Source: CAD feature listing. Evaluate the final solid. Frame: model axes, mm. Face numbers are marked on the shaded views. A direction names the side the tool comes from. Round coordinates to 2 decimals unless told otherwise and drop trailing zeros. Loops run counter-clockwise (first coordinate to the right, second up) from the corner with the lowest first, then second, coordinate; pieces in that order, holes last.
(1) Mould query, pull axis Y, two halves, no side actions, for the marked faces 6, 7 and 8. Classes: pulls with the +Y half, pulls with the -Y half, needs draft (parallel to the pull), parting line crosses it, or undercut.
(2) Material intervals for probe 1 along Y at (x, z) = (-13, 1.25); probe 2 along Y at (x, z) = (9, -4.75); probe 3 along Z at (x, y) = (-5.75, 30.5), sorted ascending.
(3) First-contact query: pin 1 Ø5 at (x, z) = (0.5, -4.5) entering from +Y; pin 2 Ø2 at (x, y) = (7.5, 8) entering from -Z; pin 3 Ø10 at (x, y) = (2.5, -23) entering from +Z; pin 4 Ø3 at (y, z) = (-10.5, -4) entering from -X. Flat tips, straight axial feed; report the tip coordinate or a pass-through.
(4) Section C-C, the plane x = -0.5. Return the cut outline in (y, z), plus the area to 3 significant figures.
(5) Set-up query: the marked faces 1, 2, 3, 4 and 5. Return all of +Z, -Z, +X, -X, +Y, -Y with unobstructed straight access to the full face (end or side cutting, diameter ignored); none if empty.
(6) Section A-A, the plane z = -2.25. Return the cut outline in (x, y) (3 decimals), plus the area to 3 significant figures.
(7) Section B-B, the plane y = -22.5. Return the cut outline in (x, z) (3 decimals), plus the area to 3 significant figures.
```python
from build123d import *

# Parameters (mm, degrees)
SKETCH_1_R           = 1
EXTRUDE_1_DEPTH      = 1.6
SKETCH_2_W           = 16.45
SKETCH_2_H           = 15.2
SKETCH_2_W_2         = 13.91
EXTRUDE_2_DEPTH      = 9.2
CUT_EXTRUDE_START    = 32.7
CUT_EXTRUDE_1_DEPTH  = 15.2
CUT_EXTRUDE_START_2  = -27.7
CUT_EXTRUDE_2_DEPTH  = 15.2
SKETCH_6_W           = 13
SKETCH_6_H           = 1.6
CUT_EXTRUDE_3_DEPTH  = 9
SKETCH_7_W           = 10.46
SKETCH_7_H           = 1.6
CUT_EXTRUDE_8_DEPTH  = 9
EXTRUDE_START        = 17.5
SKETCH_10_W          = 18.99
SKETCH_10_H          = 9.2
EXTRUDE_5_DEPTH      = 15.2
EXTRUDE_START_2      = -12.5
SKETCH_11_W          = 18.99
SKETCH_11_H          = 9.2
EXTRUDE_6_DEPTH      = 15.2
CUT_EXTRUDE_9_DEPTH  = 60.4
SKETCH_14_W          = 15.54
SKETCH_14_H          = 1.6
CUT_EXTRUDE_10_DEPTH = 9
SKETCH_15_W          = 15.54
SKETCH_15_H          = 1.6
CUT_EXTRUDE_11_DEPTH = 9


with BuildPart() as part:
    # 草图1 → 凸台-拉伸1 (new body)
    with BuildSketch(Plane.XY):
        with BuildLine():
            Line((-13, 22.5), (13, 22.5))
            ThreePointArc((13, 22.5), (14.414213562, 21.914213562), (15, 20.5))
            Line((15, 20.5), (15, -15.5))
            ThreePointArc((15, -15.5), (14.414213562, -16.914213562), (13, -17.5))
            Line((13, -17.5), (-13, -17.5))
            ThreePointArc((-13, -17.5), (-14.414213562, -16.914213562), (-15, -15.5))
            Line((-15, -15.5), (-15, 20.5))
            ThreePointArc((-15, 20.5), (-14.414213562, 21.914213562), (-13, 22.5))
        make_face()
        with Locations((-13, 20.5)):
            Circle(SKETCH_1_R, mode=Mode.SUBTRACT)
        with Locations((13, 20.5)):
            Circle(SKETCH_1_R, mode=Mode.SUBTRACT)
        with Locations((13, -15.5)):
            Circle(SKETCH_1_R, mode=Mode.SUBTRACT)
        with Locations((-13, -15.5)):
            Circle(SKETCH_1_R, mode=Mode.SUBTRACT)
    extrude(amount=EXTRUDE_1_DEPTH)

    # 草图2 → 凸台-拉伸2 (add)
    with BuildSketch(Plane.XY):
        with Locations((0, 25.1)):
            Rectangle(SKETCH_2_W, SKETCH_2_H)
        with Locations((0, -20.1)):
            Rectangle(SKETCH_2_W_2, SKETCH_2_H)
    extrude(amount=-EXTRUDE_2_DEPTH)

    # 草图3 → 切除-拉伸1 (cut)
    with BuildSketch(Plane(origin=(0, 0, 0), x_dir=(1, 0, 0), z_dir=(0, 1, 0)).offset(CUT_EXTRUDE_START)):
        Polygon((-8.225, 9.2), (-7.225, 9.2), (-8.225, 8.2), align=None)
        Polygon((-8.225, 0), (-7.225, 0), (-8.225, 1), align=None)
        Polygon((8.225, 0), (8.225, 1), (7.225, 0), align=None)
        Polygon((8.225, 9.2), (7.225, 9.2), (8.225, 8.2), align=None)
    extrude(amount=-CUT_EXTRUDE_1_DEPTH, mode=Mode.SUBTRACT)

    # 草图4 → 切除-拉伸2 (cut)
    with BuildSketch(Plane(origin=(0, 0, 0), x_dir=(1, 0, 0), z_dir=(0, 1, 0)).offset(CUT_EXTRUDE_START_2)):
        Polygon((-6.955, 0), (-5.955, 0), (-6.955, 1), align=None)
        Polygon((-6.955, 9.2), (-6.955, 8.2), (-5.955, 9.2), align=None)
        Polygon((6.955, 0), (6.955, 1), (5.955, 0), align=None)
        Polygon((6.955, 9.2), (6.955, 8.2), (5.955, 9.2), align=None)
    extrude(amount=CUT_EXTRUDE_2_DEPTH, mode=Mode.SUBTRACT)

    # 草图6 → 切除-拉伸3 (cut)
    with BuildSketch(Plane(origin=(0, 0, 0), x_dir=(1, 0, 0), z_dir=(0, 1, 0)).offset(CUT_EXTRUDE_START)):
        with Locations((0, 4.6)):
            Rectangle(SKETCH_6_W, SKETCH_6_H)
    extrude(amount=-CUT_EXTRUDE_3_DEPTH, mode=Mode.SUBTRACT)

    # 草图7 → 切除-拉伸8 (cut)
    with BuildSketch(Plane(origin=(0, 0, 0), x_dir=(1, 0, 0), z_dir=(0, 1, 0)).offset(CUT_EXTRUDE_START_2)):
        with Locations((0, 4.6)):
            Rectangle(SKETCH_7_W, SKETCH_7_H)
    extrude(amount=CUT_EXTRUDE_8_DEPTH, mode=Mode.SUBTRACT)

    # 草图10 → 凸台-拉伸5 (add)
    with BuildSketch(Plane(origin=(0, 0, 0), x_dir=(1, 0, 0), z_dir=(0, 1, 0)).offset(EXTRUDE_START)):
        with Locations((0, 4.6)):
            Rectangle(SKETCH_10_W, SKETCH_10_H)
    extrude(amount=EXTRUDE_5_DEPTH)

    # 草图11 → 凸台-拉伸6 (add)
    with BuildSketch(Plane(origin=(0, 0, 0), x_dir=(1, 0, 0), z_dir=(0, 1, 0)).offset(EXTRUDE_START_2)):
        with Locations((0, 4.6)):
            Rectangle(SKETCH_11_W, SKETCH_11_H)
    extrude(amount=-EXTRUDE_6_DEPTH)

    # 草图12 → 切除-拉伸9 (cut)
    with BuildSketch(Plane(origin=(0, 0, 0), x_dir=(1, 0, 0), z_dir=(0, 1, 0)).offset(CUT_EXTRUDE_START)):
        Polygon((-9.495, 9.2), (-8.495, 9.2), (-9.495, 8.2), align=None)
        Polygon((-9.495, 0), (-8.495, 0), (-9.495, 1), align=None)
        Polygon((9.495, 9.2), (8.495, 9.2), (9.495, 8.2), align=None)
        Polygon((9.495, 0), (9.495, 1), (8.495, 0), align=None)
    extrude(amount=-CUT_EXTRUDE_9_DEPTH, mode=Mode.SUBTRACT)

    # 草图14 → 切除-拉伸10 (cut)
    with BuildSketch(Plane(origin=(0, 0, 0), x_dir=(1, 0, 0), z_dir=(0, 1, 0)).offset(CUT_EXTRUDE_START)):
        with Locations((0, 4.6)):
            Rectangle(SKETCH_14_W, SKETCH_14_H)
    extrude(amount=-CUT_EXTRUDE_10_DEPTH, mode=Mode.SUBTRACT)

    # 草图15 → 切除-拉伸11 (cut)
    with BuildSketch(Plane(origin=(0, 0, 0), x_dir=(1, 0, 0), z_dir=(0, 1, 0)).offset(CUT_EXTRUDE_START_2)):
        with Locations((0, 4.6)):
            Rectangle(SKETCH_15_W, SKETCH_15_H)
    extrude(amount=CUT_EXTRUDE_11_DEPTH, mode=Mode.SUBTRACT)


solid = part.part
```
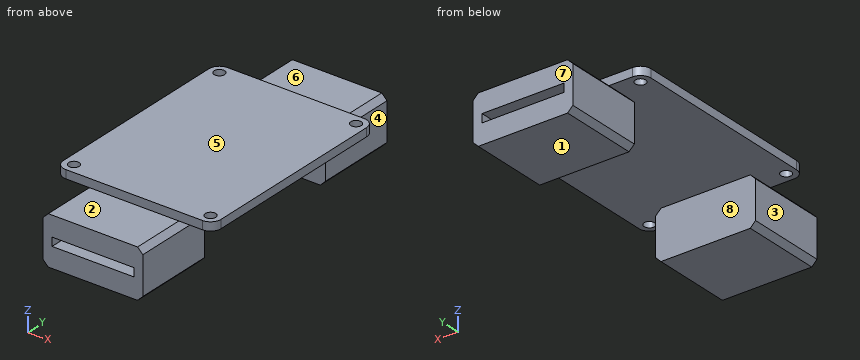
Output values:
1. face 6: needs draft
1. face 7: pulls with the +Y half
1. face 8: undercut
2. probe 1: y = -17.5 to -16.5, -14.5 to 19.5, 21.5 to 22.5
2. probe 2: y = -27.7 to -12.5, 17.5 to 32.7
2. probe 3: z = -9.2 to -5.4, -3.8 to 0
3. pin 1: stops at y = 32.7
3. pin 2: stops at z = 0
3. pin 3: stops at z = 0
3. pin 4: passes through
4. outline: (-27.7, -9.2) - (-12.5, -9.2) - (-12.5, 0) - (17.5, 0) - (17.5, -9.2) - (32.7, -9.2) - (32.7, -5.4) - (23.7, -5.4) - (23.7, -3.8) - (32.7, -3.8) - (32.7, 0) - (22.5, 0) - (22.5, 1.6) - (-17.5, 1.6) - (-17.5, 0) - (-27.7, 0) - (-27.7, -3.8) - (-18.7, -3.8) - (-18.7, -5.4) - (-27.7, -5.4) - close
4. area: 315 mm2
5. face 1: -Z, +X, -X, +Y, -Y
5. face 2: +Z, +X, -X, -Y
5. face 3: -Z, -X, +Y, -Y
5. face 4: -Z, +X, +Y, -Y
5. face 5: +Z, +X, -X, +Y, -Y
6. outline: (-9.495, -27.7) - (9.495, -27.7) - (9.495, -12.5) - (-9.495, -12.5) - close; (-9.495, 17.5) - (9.495, 17.5) - (9.495, 32.7) - (-9.495, 32.7) - close
6. area: 577 mm2
7. outline: (-9.495, -8.2) - (-8.495, -9.2) - (8.495, -9.2) - (9.495, -8.2) - (9.495, -1) - (8.495, 0) - (-8.495, 0) - (-9.495, -1) - close; hole (-7.77, -5.4) - (7.77, -5.4) - (7.77, -3.8) - (-7.77, -3.8) - close
7. area: 148 mm2
